Input: part model. Units: mm. Frame: model coordinates. A direction names the side the tool comes from. Coordinates: 2 decimals unless noted, no trailing zeros. Order: outer loops, then holes, each group sorted by start corner. A loop starts at its lowest first (then second) coordinate and runs counter-clockwise, first axis right, second up. Notation, with made-up numbers: M 24,35.5 L 68,35.5 A24 cw 68,59.5 Z; hole C 5,87.5 d8. An arc over 180 degrees is marked long. One line per item, written item: value.
```python
from build123d import *

# Parameters (mm, degrees)
BOSS_EXTRUDE1_OUTLINE_R = 3.2639
BOSS_EXTRUDE1_DEPTH     = 20.6248
SKETCH2_OUTSIDE_W       = 22.294
SKETCH2_OUTSIDE_H       = 20.332
SKETCH2_OUTSIDE_R       = 4.7625
CUT_EXTRUDE2_DEPTH      = 11.0998


# Read off the part's stored shape, not the designer's step: Boss-Extrude1
with BuildPart() as part:
    # Boss-Extrude1 outline → Boss-Extrude1 (new body)
    with BuildSketch(Plane(origin=(0, 0, 0), x_dir=(1, 0, 0), z_dir=(0, 1, 0))):
        Polygon((3.658841861, -6.3373), (7.317683722, 0), (3.658841861, 6.3373), (-3.658841861, 6.3373), (-7.317683722, 0), (-3.658841861, -6.3373), align=None)
        with Locations((0, -1.016)):
            Circle(BOSS_EXTRUDE1_OUTLINE_R, mode=Mode.SUBTRACT)
    extrude(amount=BOSS_EXTRUDE1_DEPTH)

    # Sketch2 outside → Cut-Extrude2 (cut)
    with BuildSketch(Plane(origin=(0, 20.6248, 0), x_dir=(1, 0, 0), z_dir=(0, 1, 0))):
        Rectangle(SKETCH2_OUTSIDE_W, SKETCH2_OUTSIDE_H)
        with Locations(Location((0, 0, 0), (0, 0, 270))):
            Circle(SKETCH2_OUTSIDE_R, mode=Mode.SUBTRACT)
    extrude(amount=-CUT_EXTRUDE2_DEPTH, mode=Mode.SUBTRACT)


solid = part.part
```
(1) First-contact query: pin 1 (6 mm diameter, centred on y = 9.5, z = 4, fed in from -X); pin 2 (1.5 mm diameter, centred on x = -2.5, y = 13, fed in from -Z); pin 3 (3 mm diameter, centred on x = 4.5, z = 5, fed in from +Y) (3 decimals). Flat tips, straight axial feed; report the tip coordinate or a pass-through.
Data:
pin 1: stops at x = -6.74
pin 2: stops at z = -4.43
pin 3: stops at y = 9.525
(2) Cut plane B-B on z = 3.75. Output: boundary loops of the cut face in (x, y) (3 decimals).
Data:
outline: M -5.153,0 L -1.783,0 L -1.783,20.625 L -2.936,20.625 L -2.936,9.525 L -5.153,9.525 Z; M 1.783,0 L 5.153,0 L 5.153,9.525 L 2.936,9.525 L 2.936,20.625 L 1.783,20.625 Z
(3) Cut plane A-A on x = 0. Output: boundary loops of the cut face in (y, z) (1 decimal), plus the area to 3 significant figures.
Data:
outline: M 0,-6.3 L 9.5,-6.3 L 9.5,-4.8 L 20.6,-4.8 L 20.6,-2.2 L 0,-2.2 Z; M 0,4.3 L 20.6,4.3 L 20.6,4.8 L 9.5,4.8 L 9.5,6.3 L 0,6.3 Z
area: 91.8 mm2
(4) Draft query along X for faces 3 (the flat face through (5.463, 4.696, 3.213)), 4 (the cylindrical face through (-2.59, 10.17, 3)), 5 (the flat face through (0, 5, 6.337)), 6 (the flat face through (-5.463, 4.696, -3.213)). Return one class per face: released by +X, released by -X, zero draft, split by the parting line, or undercut.
Data:
face 3: released by +X
face 4: undercut
face 5: zero draft
face 6: released by -X
(5) Ray query, line 1 (Z direction, x = 0, y = 8.5); line 2 (Z direction, x = -0.25, y = 19.5); line 3 (Y direction, x = 3.5, z = 4.25) (3 decimals). Return the intervals inside material, ascending. Write a range as from..to.
Data:
line 1: z = -6.34..-2.25, 4.28..6.34
line 2: z = -4.76..-2.24, 4.27..4.76
line 3: y = 0..9.525
(6) Cut plane C-C on y = 7. Output: boundary loops of the cut face in (x, z), plus the area to 3 significant figures.
Data:
outline: M -7.32,0 L -3.66,-6.34 L 3.66,-6.34 L 7.32,0 L 3.66,6.34 L -3.66,6.34 Z; hole C 0,1.02 d6.53
area: 106 mm2
(7) Cut plane D-D on z = -5.5. Output: boundary loops of the cut face in (x, y) (3 decimals).
Data:
outline: M -4.142,0 L 4.142,0 L 4.142,9.525 L -4.142,9.525 Z
(8) Access query for faces 1 (the flat face through (5, 9.525, 0)), 2 (the flat face through (5.514, 4.696, -3.124)). Directions: +Z, -Z, +X, -X, +Y, -Y. A direction counts if a zero-diameter tool reaches every point of the face in a straight line with its end or side. Return the directions, or none.
Data:
face 1: +Y
face 2: -Z, +X, +Y, -Y
